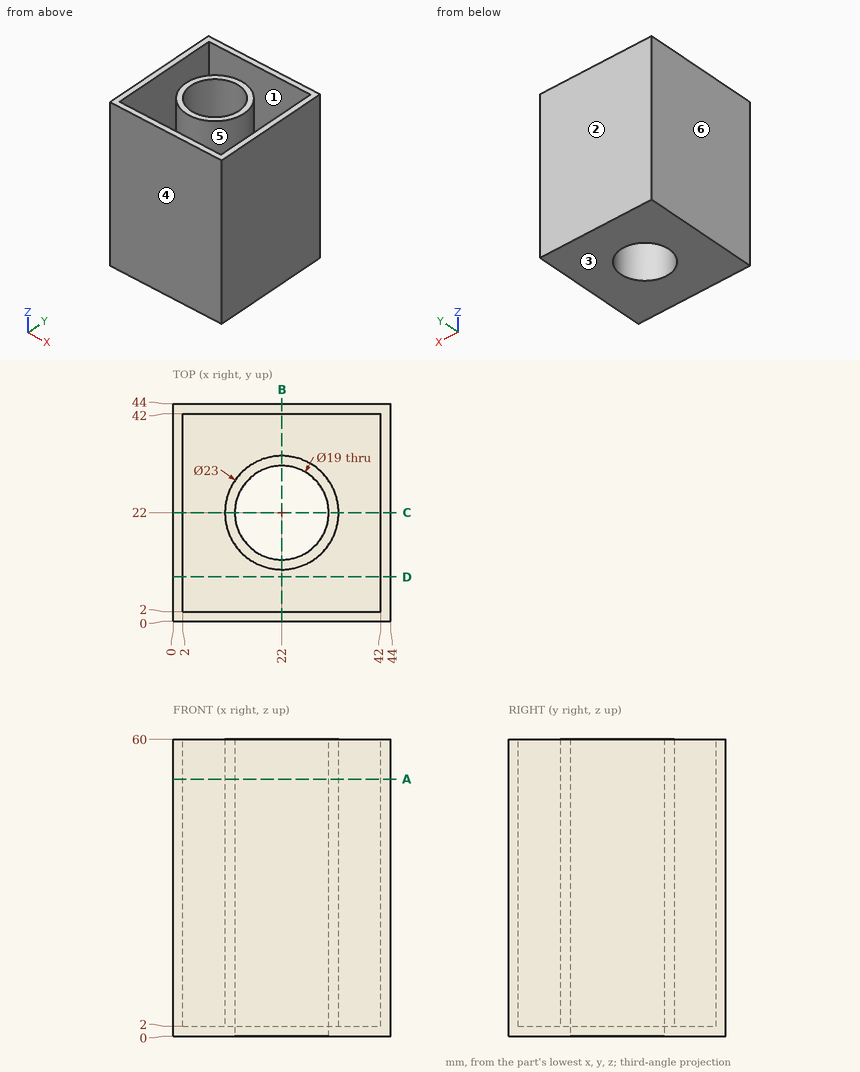
Could you check a few things on this drawing? It's one solid part, dimensions in mm from its lowest x, y, z. A direction names the side the tool comes from. Coordinates: 2 decimals unless noted, no trailing zeros. Write each loop counter-clockwise with the first axis right and the second up, starting at its lowest first coordinate (ties: lowest second). Pieces come first, ordered by that corner, then holes. Notation, with made-up numbers: (25, -1.75) - (30, -1.75) arc R34 ccw to (30, 32.25) - close; hole circle Ø7 at (71.25, 36.25). An arc over 180 degrees is marked (long way). Use one line per item in the form item = value.
1) Suppose I cut it at A-A, the plane z = 52. Write out the boundary of the cut face in (x, y), plus the area to 3 significant figures.
Solved:
outline = (0, 0) - (44, 0) - (44, 44) - (0, 44) - close; circle Ø23 at (22, 22); hole (2, 2) - (42, 2) - (42, 42) - (2, 42) - close; hole circle Ø19 at (22, 22)
area = 468 mm2
2) I'm going to push a flat-ended pin straight in: P1, Ø3, axis at x = 32.5, y = 8.5, coming from the +Z side. Where does the tip first touch, or does it pass through?
Solved:
P1 = 2
3) Suppose I cut it at B-B, the plane x = 22. Write out the boundary of the cut face in (y, z), plus the area to 3 significant figures.
Solved:
outline = (0, 0) - (12.5, 0) - (12.5, 60) - (10.5, 60) - (10.5, 2) - (2, 2) - (2, 60) - (0, 60) - close; (31.5, 0) - (44, 0) - (44, 60) - (42, 60) - (42, 2) - (33.5, 2) - (33.5, 60) - (31.5, 60) - close
area = 514 mm2
4) Thinking about a two-plate mould opening in Y: for the marked faces 1, 2, 3 and 4, which applies, released by +Y, released by -Y, zero draft, split by the parting line, or undercut?
Solved:
face_1 = undercut
face_2 = released by +Y
face_3 = zero draft
face_4 = released by -Y
5) I need wall thicknesses on line 1 (Y direction, x = 22, z = 33); line 2 (X direction, y = 35.5, z = 23); line 3 (Y direction, x = 19, z = 4.5). Which ranges of each line are inside material? Lowest first, please.
Solved:
line_1 = 0 to 2, 10.5 to 12.5, 31.5 to 33.5, 42 to 44
line_2 = 0 to 2, 42 to 44
line_3 = 0 to 2, 10.9 to 12.99, 31.01 to 33.1, 42 to 44
6) Suppose I cut it at D-D, the plane y = 9. Write out the boundary of the cut face in (x, z), plus the area to 3 significant figures.
Solved:
outline = (0, 0) - (44, 0) - (44, 60) - (42, 60) - (42, 2) - (2, 2) - (2, 60) - (0, 60) - close
area = 320 mm2
7) On a 3-axis mill with a long thin cutter (end or side, diameter ignored), from which of +Z, -Z, +X, -X, +Y, -Y can I reach the whole of each face in a straight line? I mean the marked faces 5 and 6. Say none if no direction works.
Solved:
face_5 = +Z
face_6 = +Z, -Z, -X, +Y, -Y
